Read the model definition and answer for the solid it produces. Units are mm, in the model's axes. Face numbers are marked on the shaded views. Give positions to 0.01 mm unless a question says otherwise; leave off trailing zeros. Loops run counter-clockwise (first coordinate to the right, second up) from the corner with the lowest first, then second, coordinate; pieces in that order, holes last. Notation, with made-up numbers: (23, 36.25) -> (70, 36.25) arc R31 ccw to (70, 66.25) -> close; hole circle Ø8 at (49.5, -36.75). An arc over 180 degrees is marked (long way). Write each question's results on one line, items separated by ' | '. Start each with the question number.
Item 1: Determine the mould class of the marked faces 1 and 2 for opening direction Z: +Z half, -Z half, draft (parallel to the pull), parting line (faces both ways), or undercut.
Item 2: Section A-A on x = 21.5 is taken. Write down the section's boundary in (y, z) (3 decimals).
Item 3: Each of these flat-tipped pins is pushed along its axis until it touches: P1, Ø0.8, axis at x = -7.97, z = 0, coming from the +Y side; P2, Ø0.7, axis at x = 16.5, z = 0, coming from the -Y side; P3, Ø1.1, axis at x = -15.94, z = 0, coming from the -Y side. Where does it stop, or does it pass through?
Item 4: Find the intervals of material crossed by line 1 (Z direction, x = -28.5, y = -2.75) (3 decimals); line 2 (Y direction, x = -18.5, z = 2.25); line 3 (Z direction, x = -16.5, y = -1.55) (3 decimals), in increasing order.
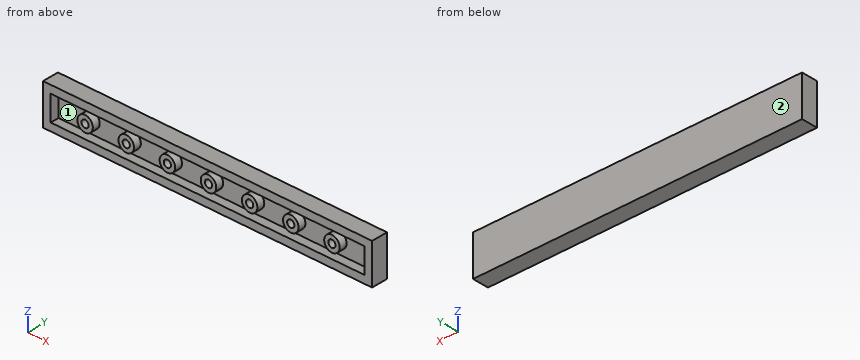
```python
from build123d import *

# Parameters (mm, degrees)
SKETCH1_W           = 63.75
SKETCH1_H           = 7.85
BOSS_EXTRUDE1_DEPTH = 3.15
SHELL1_T            = -1.5
SKETCH2_R           = 1.5
SKETCH2_R_2         = 0.7
BOSS_EXTRUDE2_DEPTH = 1.45


with BuildPart() as part:
    # Sketch1 → Boss-Extrude1 (new body)
    with BuildSketch(Plane(origin=(0, 0, 0), x_dir=(1, 0, 0), z_dir=(0, 1, 0))):
        Rectangle(SKETCH1_W, SKETCH1_H)
    extrude(amount=-BOSS_EXTRUDE1_DEPTH)

    # Shell1
    shell1_openings = [part.faces().sort_by_distance(p)[0] for p in [
        (0, -3.15, 0),
    ]]
    offset(amount=SHELL1_T, openings=shell1_openings, kind=Kind.INTERSECTION)

    # Sketch2 → Boss-Extrude2 (add)
    # profile 1 of 7: a face of its own
    with BuildSketch(Plane.XZ.offset(1.5)):
        with Locations(Location((-23.90625, 0, 0), (0, 0, 90))):
            Circle(SKETCH2_R)
        with Locations(Location((-23.90625, 0, 0), (0, 0, 90))):
            Circle(SKETCH2_R_2, mode=Mode.SUBTRACT)
    # profile 2 of 7: a face of its own
    with BuildSketch(Plane.XZ.offset(1.5)):
        with Locations(Location((-15.93625, 0, 0), (0, 0, 90))):
            Circle(SKETCH2_R)
        with Locations(Location((-15.93625, 0, 0), (0, 0, 90))):
            Circle(SKETCH2_R_2, mode=Mode.SUBTRACT)
    # profile 3 of 7: a face of its own
    with BuildSketch(Plane.XZ.offset(1.5)):
        with Locations(Location((-7.96625, 0, 0), (0, 0, 90))):
            Circle(SKETCH2_R)
        with Locations(Location((-7.96625, 0, 0), (0, 0, 90))):
            Circle(SKETCH2_R_2, mode=Mode.SUBTRACT)
    # profile 4 of 7: a face of its own
    with BuildSketch(Plane.XZ.offset(1.5)):
        with Locations(Location((0.00375, 0, 0), (0, 0, 90))):
            Circle(SKETCH2_R)
        with Locations(Location((0.00375, 0, 0), (0, 0, 90))):
            Circle(SKETCH2_R_2, mode=Mode.SUBTRACT)
    # profile 5 of 7: a face of its own
    with BuildSketch(Plane.XZ.offset(1.5)):
        with Locations(Location((7.97375, 0, 0), (0, 0, 90))):
            Circle(SKETCH2_R)
        with Locations(Location((7.97375, 0, 0), (0, 0, 90))):
            Circle(SKETCH2_R_2, mode=Mode.SUBTRACT)
    # profile 6 of 7: a face of its own
    with BuildSketch(Plane.XZ.offset(1.5)):
        with Locations(Location((15.94375, 0, 0), (0, 0, 90))):
            Circle(SKETCH2_R)
        with Locations(Location((15.94375, 0, 0), (0, 0, 90))):
            Circle(SKETCH2_R_2, mode=Mode.SUBTRACT)
    # profile 7 of 7: a face of its own
    with BuildSketch(Plane.XZ.offset(1.5)):
        with Locations(Location((23.91375, 0, 0), (0, 0, 90))):
            Circle(SKETCH2_R)
        with Locations(Location((23.91375, 0, 0), (0, 0, 90))):
            Circle(SKETCH2_R_2, mode=Mode.SUBTRACT)
    extrude(amount=BOSS_EXTRUDE2_DEPTH)


solid = part.part
```
Findings:
1) face 1: undercut | face 2: draft
2) outline: (-3.15, -3.925) -> (0, -3.925) -> (0, 3.925) -> (-3.15, 3.925) -> (-3.15, 2.425) -> (-1.5, 2.425) -> (-1.5, -2.425) -> (-3.15, -2.425) -> close
3) P1: y = 0 | P2: y = -2.95 | P3: y = -1.5
4) line 1: -3.925 to -2.425, 2.425 to 3.925 | line 2: -1.5 to 0 | line 3: -3.925 to -2.425, -1.39 to -0.415, 0.415 to 1.39, 2.425 to 3.925
